Autodesk Inventor part; units mm, degrees
ref_plane "YZ Plane" through (0, 0, 0) normal (1, 0, 0) x (0, 1, 0)
ref_plane "XZ Plane" through (0, 0, 0) normal (0, 1, 0) x (-1, 0, 0)
ref_plane "XY Plane" through (0, 0, 0) normal (0, 0, 1) x (1, 0, 0)
sketch "Sketch1" plane through (0, 0, 0) normal (0, 0, 1) x (1, 0, 0)
  line L0 (-75, 75) -> (75, -75) construction
  line L1 (75, 75) -> (-75, -75) construction
  line L2 (0, -75) -> (15.375, -75)
  line L3 (15.375, -75) -> (15.375, -69)
  line L4 (15.375, -69) -> (46.125, -69)
  line L5 (46.125, -69) -> (46.125, -75)
  line L6 (75, -75) -> (46.125, -75)
  line L7 (75, -75) -> (75, -44.25)
  line L8 (75, 0) -> (75, -15.375)
  line L9 (75, -15.375) -> (69, -15.375)
  line L10 (69, -15.375) -> (69, -46.125)
  line L11 (69, -46.125) -> (75, -46.125)
  line L12 (75, 0) -> (75, 15.375)
  line L13 (75, 15.375) -> (69, 15.375)
  line L14 (69, 15.375) -> (69, 46.125)
  line L15 (69, 46.125) -> (75, 46.125)
  line L16 (-15.375, -75) -> (-15.375, -69)
  line L17 (-15.375, -69) -> (-46.125, -69)
  line L18 (-46.125, -69) -> (-46.125, -75)
  line L19 (-75, -75) -> (-46.125, -75)
  line L20 (-75, 15.375) -> (-69, 15.375)
  line L21 (-69, 15.375) -> (-69, 46.125)
  line L22 (-69, 46.125) -> (-75, 46.125)
  line L23 (-15.375, 75) -> (-15.375, 69)
  line L24 (-15.375, 69) -> (-46.125, 69)
  line L25 (-46.125, 69) -> (-46.125, 75)
  line L26 (15.375, 75) -> (15.375, 69)
  line L27 (15.375, 69) -> (46.125, 69)
  line L28 (46.125, 69) -> (46.125, 75)
  line L29 (-69, -46.125) -> (-75, -46.125)
  line L30 (-69, -15.375) -> (-69, -46.125)
  line L31 (-75, -15.375) -> (-69, -15.375)
  line L32 (15.375, -75) -> (-15.375, -75)
  line L33 (-46.125, -75) -> (-75, -75)
  line L34 (75, 75) -> (75, 46.125)
  line L35 (75, 15.375) -> (75, -15.375)
  line L36 (75, -46.125) -> (75, -75)
  line L37 (-75, 75) -> (-46.125, 75)
  line L38 (-75, 46.125) -> (-75, 75)
  line L39 (-75, -15.375) -> (-75, 15.375)
  line L40 (-75, -46.125) -> (-75, -75)
  line L41 (-15.375, 75) -> (15.375, 75)
  line L42 (46.125, 75) -> (75, 75)
  point P0 (0, 0)
  dimension "d0" = 150
  dimension "d1" = 150
  dimension "d2" = 15.375
  dimension "d3" = 6
  dimension "d4" = 30.75
  dimension "d8" = 15.375
  dimension "d9" = 6
  dimension "d10" = 30.75
extrude "Extrusion1" add sketch "Sketch1" along normal blind 6
properties part number "Backandfront_2"
Check sheet for the modelled part. Datum: model origin and axes. Units: mm. A direction names the side the tool comes from. Round coordinates to 2 decimals unless told otherwise and drop trailing zeros. Loops run counter-clockwise (first coordinate to the right, second up) from the corner with the lowest first, then second, coordinate; pieces in that order, holes last.
1. Set-up check for faces 1 (the flat face through (-1, 1, 6)), 2 (the flat face through (-46.125, -72, 3)), 3 (the flat face through (-72, -46.125, 3)), 4 (the flat face through (31, 69, 3)): record each of +Z, -Z, +X, -X, +Y, -Y from which the full face is reachable in a straight line by a thin tool's end or side.
2. Scan line: probe 1 along Y at (x, z) = (43, 0.95). Record every from-to range of solid material in increasing order.
3. Sectioned sample at A-A on y = 17.5. Record the boundary of the cut face in (x, z).
4. Mould release check, pull along Y, two halves, no side actions. Record for faces 5 (the flat face through (72, -46.125, 3)), 6 (the flat face through (-31, -69, 3)), 7 (the flat face through (72, 46.125, 3)), 8 (the flat face through (-75, -60, 3)): released by +Y, released by -Y, zero draft, split by the parting line, or undercut.
5. Gauge pin test, flat ends, axial feed: pin 1 Ø4 at (x, y) = (2, 29.5) entering from -Z; pin 2 Ø3 at (y, z) = (-31, 2) entering from -X; pin 3 Ø3 at (x, z) = (-31, 3.5) entering from -Y; pin 4 Ø3 at (y, z) = (-24.5, 3) entering from +X. Record the tip position at first contact, or that the pin passes through.
Recorded:
1. face 1: +Z, +X, -X, +Y, -Y
1. face 2: +Z, -Z, -Y
1. face 3: +Z, -Z, -X
1. face 4: +Z, -Z, +Y
2. probe 1: y = -69 to 69
3. outline: (-69, 0) - (69, 0) - (69, 6) - (-69, 6) - close
4. face 5: undercut
4. face 6: released by -Y
4. face 7: undercut
4. face 8: zero draft
5. pin 1: stops at z = 0
5. pin 2: stops at x = -69
5. pin 3: stops at y = -69
5. pin 4: stops at x = 69
